from build123d import *

# Parameters (mm, degrees)
Y_KSEKLIK_EKSTR_ZYON1_DEPTH = 10
KES_EKSTR_ZYON1_DEPTH       = 3
IZIM4_R                     = 1.5
KES_EKSTR_ZYON2_DEPTH       = 7.5
IZIM5_W                     = 20
IZIM5_H                     = 16.82010055
KES_EKSTR_ZYON4_DEPTH       = 5.5
IZIM6_R                     = 1.5
KES_EKSTR_ZYON5_DEPTH       = 19
KES_EKSTR_ZYON6_DEPTH       = 12


with BuildPart() as part:
    # Çizim1 → Yükseklik-Ekstrüzyon1 (new, symmetric)
    with BuildSketch(Plane.XY):
        with BuildLine():
            Line((-12.5, 7.5), (57.5, 7.5))
            Line((57.5, 7.5), (57.5, -7.5))
            Line((57.5, -7.5), (-12.5, -7.5))
            ThreePointArc((-12.5, -7.5), (-20, 0), (-12.5, 7.5))
        make_face()
    extrude(amount=Y_KSEKLIK_EKSTR_ZYON1_DEPTH, both=True)

    # Çizim2 → Kes-Ekstrüzyon1 (cut, symmetric)
    with BuildSketch(Plane.XY):
        with BuildLine():
            Line((6.719945644, -7.5), (-13.280054356, -7.5))
            ThreePointArc((-13.280054356, -7.5), (-20.780054356, 0), (-13.280054356, 7.5))
            Line((-13.280054356, 7.5), (6.719945644, 7.5))
            Line((6.719945644, 7.5), (6.719945644, -7.5))
        make_face()
    extrude(amount=KES_EKSTR_ZYON1_DEPTH, both=True, mode=Mode.SUBTRACT)

    # Çizim4 → Kes-Ekstrüzyon2 (cut, symmetric)
    with BuildSketch(Plane.XY):
        with Locations((-10, 0)):
            Circle(IZIM4_R)
    extrude(amount=KES_EKSTR_ZYON2_DEPTH, both=True, mode=Mode.SUBTRACT)

    # Çizim5 → Kes-Ekstrüzyon4 (cut, symmetric)
    with BuildSketch(Plane.XY):
        with Locations((47.5, -0.910050275)):
            Rectangle(IZIM5_W, IZIM5_H)
    extrude(amount=KES_EKSTR_ZYON4_DEPTH, both=True, mode=Mode.SUBTRACT)

    # Çizim6 → Kes-Ekstrüzyon5 (cut)
    with BuildSketch(Plane.XY.offset(10)):
        with Locations((47.5, 0)):
            Circle(IZIM6_R)
    extrude(amount=-KES_EKSTR_ZYON5_DEPTH, mode=Mode.SUBTRACT)

    # Çizim7 → Kes-Ekstrüzyon6 (cut, symmetric)
    with BuildSketch(Plane(origin=(0, 0, 0), x_dir=(1, 0, 0), z_dir=(0, 1, 0))):
        Polygon((32.353261004, -10), (32.353261004, -5), (-23.403314964, -5), (-23.403314964, 5), (32.941056233, 5), (32.941056233, 10), (-29.197296503, 10), (-29.197296503, -10), align=None)
    extrude(amount=KES_EKSTR_ZYON6_DEPTH, both=True, mode=Mode.SUBTRACT)


solid = part.part
Read the model definition and answer for the solid it produces. Units are mm, in the model's axes. A direction names the side the tool comes from. Round coordinates to 2 decimals unless told otherwise and drop trailing zeros. Order: outer loops, then holes, each group sorted by start corner. A loop starts at its lowest first (then second) coordinate and runs counter-clockwise, first axis right, second up. Notation, with made-up numbers: (60, -26.75) - (69, -26.75) arc R20 ccw to (69, -7.75) - close; hole circle Ø1 at (-5.75, 70). An arc over 180 degrees is marked (long way). Use one line per item in the form item = value. Start each with the question number.
(1) Flat-ended cylindrical pins translate along their axes: pin 1 Ø1.5 at (y, z) = (2.5, -8.5) entering from -X; pin 2 Ø0.9 at (x, y) = (48, 0) entering from +Z; pin 3 Ø7.5 at (x, y) = (-2.5, -0.5) entering from -Z. Find the tip coordinate at first contact, or state that the pin passes through.
(2) The part is cut by section C-C (z = 8.75). Give the vertices of the cut face in (x, y), then the cut area to 3 significant figures.
(3) Find the intervals of material crossed by line 1 along Y through (x, z) = (47.5, -8.15); line 2 along Z through (x, y) = (-8.5, 0.75); line 3 along Z through (x, y) = (8.5, -4), in increasing order. Write a range as from..to.
(4) For faces 4 (the face through (46, 0, 8)), 5 (the face through (-6, 0, 3)), 6 (the face through (32.941, 0, -7)), 7 (the face through (47, 2, 5.5)), 8 (the face through (7, 0, 5)), determine the directions among +Z, -Z, +X, -X, +Y, -Y from which every point of the face is accessible in a straight line to the end or side of a thin tool.
(5) The part is cut by section D-D (x = -10). Give the vertices of the cut face in (y, z), then the cut area to 3 significant figures.
(6) Determine the mould class of faces 1 (the face through (-11.5, 0.07, -3.99)), 2 (the face through (37.5, 0, 0)), 3 (the face through (30, 7.5, 0)) for opening direction X: +X half, -X half, draft (parallel to the pull), parting line (faces both ways), or undercut.
(7) The part is cut by section B-B (y = 0). Count the separate pieces of the cut face and the enclosed holes in it, then the cut area to 3 significant figures.
(8) The part is cut by section A-A (x = 47.5). Give the vertices of the cut face in (y, z).
Checked values:
q1.pin_1 = 32.94
q1.pin_2 = -9
q1.pin_3 = -5
q2.outline = (32.35, -7.5) - (57.5, -7.5) - (57.5, 7.5) - (32.35, 7.5) - close; hole circle Ø3 at (47.5, 0)
q2.area = 370 mm^2
q3.line_1 = -7.5..-1.5, 1.5..7.5
q3.line_2 = -5..-3, 3..5
q3.line_3 = -5..5
q4.face_4 = +Z
q4.face_5 = -X, +Y, -Y
q4.face_6 = -Z, -X, +Y, -Y
q4.face_7 = +X, +Y, -Y
q4.face_8 = +Z, -X, +Y, -Y
q5.outline = (-7.5, -5) - (-1.5, -5) - (-1.5, -3) - (-7.5, -3) - close; (-7.5, 3) - (-1.5, 3) - (-1.5, 5) - (-7.5, 5) - close; (1.5, -5) - (7.5, -5) - (7.5, -3) - (1.5, -3) - close; (1.5, 3) - (7.5, 3) - (7.5, 5) - (1.5, 5) - close
q5.area = 48.0 mm^2
q6.face_1 = undercut
q6.face_2 = +X half
q6.face_3 = draft
q7.separate_pieces = 4
q7.enclosed_holes = 0
q7.area = 607 mm^2
q8.outline = (-7.5, -10) - (7.5, -10) - (7.5, -5.5) - (1.5, -5.5) - (1.5, -9) - (-1.5, -9) - (-1.5, -5.5) - (-7.5, -5.5) - close; (-7.5, 5.5) - (-1.5, 5.5) - (-1.5, 10) - (-7.5, 10) - close; (1.5, 5.5) - (7.5, 5.5) - (7.5, 10) - (1.5, 10) - close
